```python
from build123d import *

# Parameters (mm, degrees)
SKETCH1_W           = 200
SKETCH1_H           = 26
BOSS_EXTRUDE1_DEPTH = 25
SHELL1_T            = -3
SKETCH2_R           = 12.45
CUT_EXTRUDE1_DEPTH  = 25


with BuildPart() as part:
    # Sketch1 → Boss-Extrude1 (new body)
    with BuildSketch(Plane(origin=(0, 0, 0), x_dir=(1, 0, 0), z_dir=(0, 1, 0))):
        Rectangle(SKETCH1_W, SKETCH1_H)
    extrude(amount=BOSS_EXTRUDE1_DEPTH)

    # Shell1
    shell1_openings = [part.faces().sort_by_distance(p)[0] for p in [
        (100, 12.5, 0),
        (-100, 12.5, 0),
    ]]
    offset(amount=SHELL1_T, openings=shell1_openings, kind=Kind.INTERSECTION)

    # Sketch2 → Cut-Extrude1 (cut)
    with BuildSketch(Plane(origin=(0, 25, 0), x_dir=(1, 0, 0), z_dir=(0, 1, 0))):
        with Locations((-55, 0)):
            Circle(SKETCH2_R)
        with Locations((55, 0)):
            Circle(SKETCH2_R)
    extrude(amount=-CUT_EXTRUDE1_DEPTH, mode=Mode.SUBTRACT)


solid = part.part
```
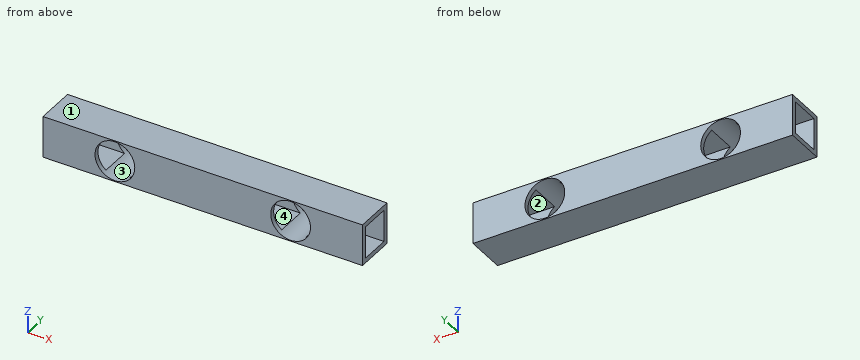
Geometry check sheet. Reference: the model listing, model coordinates, mm. Face numbers are marked on the shaded views. A direction names the side the tool comes from. Coordinates: 2 decimals unless noted, no trailing zeros. Order: outer loops, then holes, each group sorted by start corner. A loop starts at its lowest first (then second) coordinate and runs counter-clockwise, first axis right, second up. Notation, with made-up numbers: (71.5, -36) - (128.5, -36) arc R19 cw to (128.5, -19) - close; hole circle Ø2 at (-21.75, 46). An arc over 180 degrees is marked (long way). Answer in a Markdown table with one row per item. Add a question column.
1. Section check D-D (z = 0). Enter the section's corners in (x, y), plus the area to 3 significant figures.
2. Gauge pin test, flat ends, axial feed: pin 1 Ø10 at (x, z) = (89, -4) entering from -Y; pin 2 Ø15 at (x, z) = (55, 0) entering from -Y. Record the tip position at first contact, or that the pin passes through.
3. Draft check along X on the marked faces 3 and 4. Enter one of: +X half, -X half, draft (parallel to the pull), parting line (faces both ways), or undercut.
4. Section check A-A (x = -55). Enter the section's corners in (y, z), plus the area to 3 significant figures.
5. Section check B-B (y = 5). Enter the section's corners in (x, z).
6. Access from +Z, -Z, +X, -X, +Y, -Y to the whole of each face (thin tool, end or side, straight path). Record for the marked faces 1 and 2.
7. Section check C-C (x = -79.5). Enter the section's corners in (y, z).
8. Material ranges on L1, parallel to Z at x = -88.5, y = 5.25; L2, parallel to Y at x = 79.5, z = 3; L3, parallel to X at y = 20, z = -10.5, recorded low to high. Write a range as [from, to].
Data:
| question | item | result |
|---|---|---|
| 1 | outline | (-100, 0) - (-67.45, 0) - (-67.45, 3) - (-100, 3) - close; (-100, 22) - (-67.45, 22) - (-67.45, 25) - (-100, 25) - close; (-42.55, 0) - (42.55, 0) - (42.55, 3) - (-42.55, 3) - close; (-42.55, 22) - (42.55, 22) - (42.55, 25) - (-42.55, 25) - close; (67.45, 0) - (100, 0) - (100, 3) - (67.45, 3) - close; (67.45, 22) - (100, 22) - (100, 25) - (67.45, 25) - close |
| 1 | area | 901 mm² |
| 2 | pin 1 | stops at y = 0 |
| 2 | pin 2 | passes through |
| 3 | face 3 | undercut |
| 3 | face 4 | draft |
| 4 | outline | (0, -13) - (25, -13) - (25, -12.45) - (0, -12.45) - close; (0, 12.45) - (25, 12.45) - (25, 13) - (0, 13) - close |
| 4 | area | 27.5 mm² |
| 5 | outline | (-100, -13) - (100, -13) - (100, -10) - (62.42, -10) arc R12.45 cw to (47.58, -10) - (-47.58, -10) arc R12.45 cw to (-62.42, -10) - (-100, -10) - close; (-100, 10) - (-62.42, 10) arc R12.45 cw to (-47.58, 10) - (47.58, 10) arc R12.45 cw to (62.42, 10) - (100, 10) - (100, 13) - (-100, 13) - close |
| 6 | face 1 | +Z, +X, -X, +Y, -Y |
| 6 | face 2 | +X, -X |
| 7 | outline | (0, -13) - (25, -13) - (25, 13) - (0, 13) - close; hole (3, -10) - (22, -10) - (22, 10) - (3, 10) - close |
| 8 | L1 | z = [-13, -10], [10, 13] |
| 8 | L2 | y = [0, 3], [22, 25] |
| 8 | L3 | x = [-100, -61.69], [-48.31, 48.31], [61.69, 100] |
